Model file for the job. Use its own axes, mm. A direction names the side the tool comes from. Round coordinates to 2 decimals unless told otherwise and drop trailing zeros. Loops run counter-clockwise (first coordinate to the right, second up) from the corner with the lowest first, then second, coordinate; pieces in that order, holes last.
from build123d import *

# Parameters (mm, degrees)
SKETCH1_W               = 60
SKETCH1_H               = 60
SKETCH1_R               = 2.5
BOSS_EXTRUDE2_DEPTH     = 5
SKETCH3_W               = 35
SKETCH3_H               = 20
BOSS_EXTRUDE3_DEPTH     = 5
SKETCH5_R               = 2.5
CUT_EXTRUDE1_DEPTH      = 113.472218792
FILLET1_R               = 10
FILLET2_R               = 10
FILLET3_R               = 10
CUT_EXTRUDE2_DEPTH      = 113.472218792
CUT_EXTRUDE2_DEPTH_BACK = 113.472218792
SKETCH6_W               = 130
SKETCH6_H               = 2
CUT_EXTRUDE4_DEPTH      = 113.401067611
CUT_EXTRUDE4_DEPTH_BACK = 113.401067611
FILLET4_R               = 5
SKETCH8_W               = 11
SKETCH8_H               = 5
BOSS_EXTRUDE4_DEPTH     = 3
SKETCH9_W               = 11
SKETCH9_H               = 3
BOSS_EXTRUDE5_DEPTH     = 15
BOSS_EXTRUDE6_DEPTH     = 21
CUT_EXTRUDE5_DEPTH      = 93.926839714
CUT_EXTRUDE5_DEPTH_BACK = 10
SKETCH11_R              = 1.25
FILLET5_R               = 3


with BuildPart() as part:
    # Sketch1 → Boss-Extrude2 (new body)
    with BuildSketch(Plane(origin=(0, 0, 0), x_dir=(1, 0, 0), z_dir=(0, 1, 0))):
        with Locations((30, 30)):
            Rectangle(SKETCH1_W, SKETCH1_H)
        with Locations(Location((30, 40.020691429, 0), (0, 0, 270))):
            Circle(SKETCH1_R, mode=Mode.SUBTRACT)
        with Locations(Location((20, 30.020691429, 0), (0, 0, 270))):
            Circle(SKETCH1_R, mode=Mode.SUBTRACT)
        with Locations(Location((30, 20.020691429, 0), (0, 0, 270))):
            Circle(SKETCH1_R, mode=Mode.SUBTRACT)
        with Locations(Location((40, 30.020691429, 0), (0, 0, 270))):
            Circle(SKETCH1_R, mode=Mode.SUBTRACT)
        with Locations(Location((30, 30.020691429, 0), (0, 0, 270))):
            Circle(SKETCH1_R, mode=Mode.SUBTRACT)
    extrude(amount=BOSS_EXTRUDE2_DEPTH)

    # Sketch3 → Boss-Extrude3 (add)
    with BuildSketch(Plane(origin=(0, 0, 0), x_dir=(1, 0, 0), z_dir=(0, 1, 0))):
        with Locations((77.5, 30.020691429)):
            Rectangle(SKETCH3_W, SKETCH3_H)
        with Locations((-17.5, 30.020691429)):
            Rectangle(SKETCH3_W, SKETCH3_H)
    extrude(amount=BOSS_EXTRUDE3_DEPTH)

    # Sketch5 → Cut-Extrude1 (cut, through all)
    with BuildSketch(Plane(origin=(0, 0, 0), x_dir=(1, 0, 0), z_dir=(0, 1, 0))):
        with Locations(Location((70, 30.020691429, 0), (0, 0, 270))):
            Circle(SKETCH5_R)
        with Locations(Location((-10, 30.020691429, 0), (0, 0, 270))):
            Circle(SKETCH5_R)
    extrude(amount=CUT_EXTRUDE1_DEPTH, mode=Mode.SUBTRACT)

    # Fillet1
    fillet1_edges = [part.edges().sort_by_distance(p)[0] for p in [
        (95, 2.5, -20.020691429),
        (95, 2.5, -40.020691429),
    ]]
    fillet(fillet1_edges, radius=FILLET1_R - 0.0001)  # a hair under: the kernel refuses the full size

    # Fillet2
    fillet2_edges = [part.edges().sort_by_distance(p)[0] for p in [
        (-35, 2.5, -20.020691429),
        (-35, 2.5, -40.020691429),
    ]]
    fillet(fillet2_edges, radius=FILLET2_R - 0.0001)  # a hair under: the kernel refuses the full size

    # Fillet3
    fillet3_edges = [part.edges().sort_by_distance(p)[0] for p in [
        (0, 2.5, -60),
        (60, 2.5, -60),
        (60, 2.5, 0),
        (0, 2.5, 0),
    ]]
    fillet(fillet3_edges, radius=FILLET3_R)

    # Sketch6 → Cut-Extrude2 (cut, two sides: drawn at the far end of the back side and taken through both)
    with BuildSketch(Plane(origin=(0, 0, -60), x_dir=(-1, 0, 0), z_dir=(0, 0, -1)).offset(-CUT_EXTRUDE2_DEPTH_BACK)):
        with Locations((-30, 4)):
            Rectangle(SKETCH6_W, SKETCH6_H)
    extrude(amount=CUT_EXTRUDE2_DEPTH + CUT_EXTRUDE2_DEPTH_BACK, mode=Mode.SUBTRACT)

    # Sketch7 → Cut-Extrude4 (cut, two sides: drawn at the far end of the back side and taken through both)
    with BuildSketch(Plane(origin=(0, 3, 0), x_dir=(1, 0, 0), z_dir=(0, 1, 0)).offset(-CUT_EXTRUDE4_DEPTH_BACK)):
        Polygon((-16, 40.020691429), (-16, 42.339149427), (-38.923164287, 42.339149427), (-38.923164287, 39.725242292), (-38.923164287, 20.020691429), (-16, 20.020691429), align=None)
        Polygon((98.923164287, 20.020691429), (98.923164287, 39.725242292), (98.923164287, 44.006554538), (76, 44.006554538), (76, 40.020691429), (76, 20.020691429), align=None)
    extrude(amount=CUT_EXTRUDE4_DEPTH + CUT_EXTRUDE4_DEPTH_BACK, mode=Mode.SUBTRACT)

    # Fillet4
    fillet4_edges = [part.edges().sort_by_distance(p)[0] for p in [
        (-16, 1.5, -20.020691429),
        (-16, 1.5, -40.020691429),
        (76, 1.5, -40.020691429),
        (76, 1.5, -20.020691429),
    ]]
    fillet(fillet4_edges, radius=FILLET4_R)

    # Sketch8 → Boss-Extrude4 (add)
    with BuildSketch(Plane(origin=(0, 0, -40.020691429), x_dir=(-1, 0, 0), z_dir=(0, 0, -1))):
        with Locations((5.5, 5.5)):
            Rectangle(SKETCH8_W, SKETCH8_H)
    extrude(amount=-BOSS_EXTRUDE4_DEPTH)

    # Sketch9 → Boss-Extrude5 (add)
    with BuildSketch(Plane(origin=(0, 0, -40.020691429), x_dir=(-1, 0, 0), z_dir=(0, 0, -1))):
        with Locations((5.5, 6.5)):
            Rectangle(SKETCH9_W, SKETCH9_H)
    extrude(amount=BOSS_EXTRUDE5_DEPTH)

    # Sketch10 → Boss-Extrude6 (add)
    with BuildSketch(Plane.XZ.offset(-5)):
        Polygon((-25.480214152, -51.023499873), (-25.480214152, -55.020691429), (-11, -55.020691429), (0, -55.020691429), (0, -51.023499873), align=None)
    extrude(amount=BOSS_EXTRUDE6_DEPTH)

    # Sketch11 → Cut-Extrude5 (cut, two sides: drawn at the far end of the back side and taken through both)
    with BuildSketch(Plane.XY.offset(-51.023499873).offset(-CUT_EXTRUDE5_DEPTH_BACK)):
        with Locations(Location((-22.880182159, -0.931652135, 0), (0, 0, 180))):
            Circle(SKETCH11_R)
        with Locations(Location((-22.880182159, -10.431652135, 0), (0, 0, 180))):
            Circle(SKETCH11_R)
    extrude(amount=CUT_EXTRUDE5_DEPTH + CUT_EXTRUDE5_DEPTH_BACK, mode=Mode.SUBTRACT)

    # Fillet5
    fillet5_edges = [part.edges().sort_by_distance(p)[0] for p in [
        (-5.5, 8, -37.020691429),
        (-5.5, 8, -55.020691429),
        (0, -16, -53.022095651),
        (-25.480214152, 5, -53.022095651),
        (-25.480214152, -16, -53.022095651),
    ]]
    fillet(fillet5_edges, radius=FILLET5_R)


solid = part.part
Q1. Pull direction Z, two halves, no side cores. Call faces 4 (the face through (56.99, 1.52, -57.15)), 5 (the face through (-5, 5, -45)), 6 (the face through (29, 0, -24)), 7 (the face through (30, 1, 0)): pulls with the +Z half, pulls with the -Z half, needs draft (parallel to the pull), parting line crosses it, or undercut.
Q2. Tool access for faces 1 (the face through (-9.89, 1.48, -32.52)), 2 (the face through (0, 1, -15)), 3 (the face through (-5, 4, -37.021)): list every direction of +Z, -Z, +X, -X, +Y, -Y with a clear straight run to the whole face (end or side of a thin tool).
Q3. Slice it at B-B on x = 70. Give the cut face in (y, z), plus the area to 3 significant figures.
Q4. Slice it at C-C on z = -19. Give the cut face in (x, y).
Q5. Slice it at D-D on z = -41.5. Give the cut face in (x, y), plus the area to 3 significant figures.
Q6. Probe line 1 (Z direction, x = 30, y = 2.3); line 2 (Z direction, x = 70, y = 2); line 3 (Z direction, x = -11.5, y = 3.5). List the from-to ranges inside material, lowest first.
Q7. Flat gauge pins, fed straight in: P1, Ø9, axis at y = 2.5, z = -42.5, coming from the +X side; P2, Ø4.5, axis at x = -14, z = -53, coming from the +Y side; P3, Ø2, axis at x = -4.5, y = 3.5, coming from the +Z side; P4, Ø4.5, axis at x = -10, z = -30.02, coming from the +Y side. Where does each tip first touch, or does it go through?
Q8. Slice it at A-A on x = 30. Give the cut face in (y, z).
Reply:
1. face 4: pulls with the -Z half
1. face 5: undercut
1. face 6: needs draft
1. face 7: pulls with the +Z half
2. face 1: +Y, -Y
2. face 2: +Z, -X, +Y, -Y
2. face 3: +Z, +X, -X, +Y
3. outline: (0, -40.02) - (3, -40.02) - (3, -32.52) - (0, -32.52) - close; (0, -27.52) - (3, -27.52) - (3, -20.02) - (0, -20.02) - close
3. area: 45.0 mm2
4. outline: (0, 0) - (27.72, 0) - (27.72, 3) - (0, 3) - close; (32.28, 0) - (60, 0) - (60, 3) - (32.28, 3) - close
5. outline: (-11, 5) - (0, 5) - (0, 8) - (-11, 8) - close; (0, 0) - (27.98, 0) - (27.98, 3) - (0, 3) - close; (32.02, 0) - (60, 0) - (60, 3) - (32.02, 3) - close
5. area: 201 mm2
6. line 1: z = -60 to -42.52, -37.52 to -32.52, -27.52 to -22.52, -17.52 to 0
6. line 2: z = -40.02 to -32.52, -27.52 to -20.02
6. line 3: z = -55.02 to -51.02
7. P1: stops at x = 75.02
7. P2: stops at y = 5
7. P3: stops at z = -20.02
7. P4: passes through
8. outline: (0, -60) - (3, -60) - (3, -42.52) - (0, -42.52) - close; (0, -37.52) - (3, -37.52) - (3, -32.52) - (0, -32.52) - close; (0, -27.52) - (3, -27.52) - (3, -22.52) - (0, -22.52) - close; (0, -17.52) - (3, -17.52) - (3, 0) - (0, 0) - close
